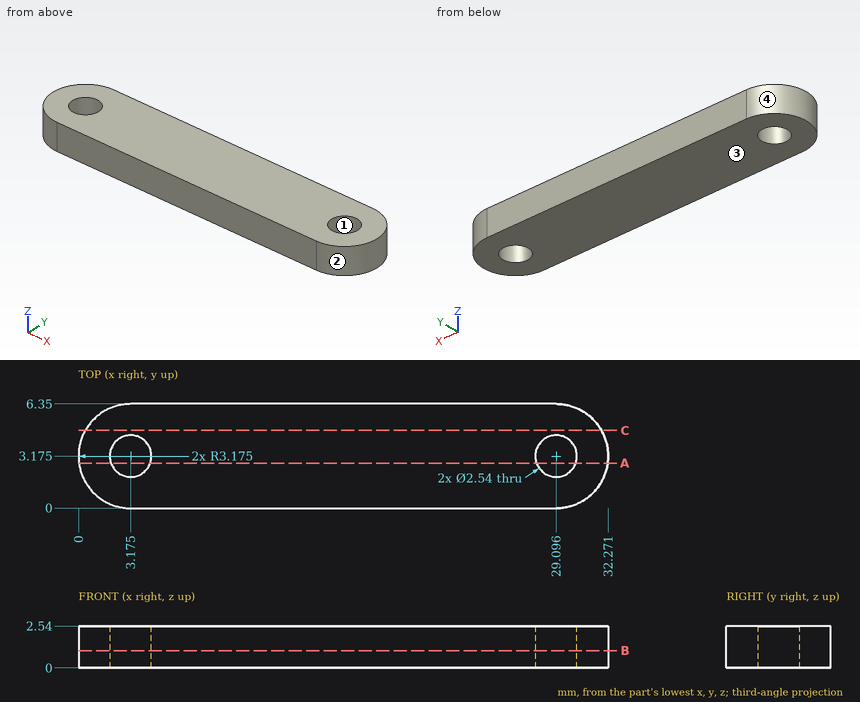
Input: dimensioned drawing with shaded views. Units: mm. Origin: part minimum x, y, z. Round coordinates to 2 decimals unless told otherwise and drop trailing zeros. Order: outer loops, then holes, each group sorted by start corner. A loop starts at its lowest first (then second) coordinate and runs counter-clockwise, first axis right, second up. Notation, with made-up numbers: M 19.5,-39.5 L 47.5,-39.5 A17 ccw 47.5,-31.5 Z; hole C -17.75,9 d4. An arc over 180 degrees is marked long. Use one line per item in the form item = value. Start each with the question number.
Q1. Cut plane C-C (y = 4.75). Return loops of the section in (x, z).
Q2. Cut plane A-A (y = 2.75). Return loops of the section in (x, z).
Q3. Mould query, pull axis X, two halves, no side actions, for the marked faces 1, 2, 3 and 4. Classes: +X half, -X half, draft (parallel to the pull), parting line (faces both ways), or undercut.
Q4. Material intervals for line 1 (X direction, y = 3, z = 0.5) (1 decimal); line 2 (X direction, y = 2.75, z = 1.2); line 3 (Y direction, x = 29, z = 1.6), sorted ascending. Write a range as [from, to].
Q5. Cut plane B-B (z = 1.05). Count the separate pieces of the cut face and the enclosed holes in it, and give its area (3 significant figures).
Geometry results:
q1.outline = M 0.42,0 L 31.85,0 L 31.85,2.54 L 0.42,2.54 Z
q2.outline = M 0.03,0 L 1.98,0 L 1.98,2.54 L 0.03,2.54 Z; M 4.37,0 L 27.9,0 L 27.9,2.54 L 4.37,2.54 Z; M 30.29,0 L 32.24,0 L 32.24,2.54 L 30.29,2.54 Z
q3.face_1 = undercut
q3.face_2 = +X half
q3.face_3 = draft
q3.face_4 = -X half
q4.line_1 = [0, 1.9], [4.4, 27.8], [30.4, 32.3]
q4.line_2 = [0.03, 1.98], [4.37, 27.9], [30.29, 32.24]
q4.line_3 = [0, 1.91], [4.44, 6.35]
q5.separate_pieces = 1
q5.enclosed_holes = 2
q5.area = 186 mm^2
